```python
from build123d import *

# Parameters (mm, degrees)
CROQUIS1_W              = 480
CROQUIS1_H              = 310
CROQUIS1_W_2            = 28
CROQUIS1_H_2            = 12
CROQUIS1_H_3            = 11
CROQUIS1_W_3            = 41.3
CROQUIS1_H_4            = 41.3
SALIENTE_EXTRUIR1_DEPTH = 12
SKETCH1_R               = 1.5
CUT_EXTRUDE1_DEPTH      = 572.527777103
SKETCH2_R               = 1.55
CUT_EXTRUDE2_DEPTH      = 12
FILLET1_R               = 5
SKETCH3_R               = 1.55
CUT_EXTRUDE3_DEPTH      = 12
BOSS_EXTRUDE1_DEPTH     = 12
FILLET2_R               = 5


with BuildPart() as part:
    # Croquis1 → Saliente-Extruir1 (new body)
    with BuildSketch(Plane(origin=(0, 0, 0), x_dir=(0, 0, -1), z_dir=(1, 0, 0))):
        with Locations((240, -155)):
            Rectangle(CROQUIS1_W, CROQUIS1_H)
        Polygon((30, -30), (450, -30), (450, -114.35), (388.7, -114.35), (388.7, -195.65), (450, -195.65), (450, -280), (30, -280), (30, -181), (70, -181), (70, -161), (30, -161), (30, -149), (70, -149), (70, -129), (30, -129), align=None, mode=Mode.SUBTRACT)
        with Locations((288, -295)):
            Rectangle(CROQUIS1_W_2, CROQUIS1_H_2, mode=Mode.SUBTRACT)
        with Locations((240, -294.5)):
            Rectangle(CROQUIS1_W_2, CROQUIS1_H_3, mode=Mode.SUBTRACT)
        with Locations((192, -295)):
            Rectangle(CROQUIS1_W_2, CROQUIS1_H_2, mode=Mode.SUBTRACT)
        with Locations((192, -15)):
            Rectangle(CROQUIS1_W_2, CROQUIS1_H_2, mode=Mode.SUBTRACT)
        with Locations((288, -15)):
            Rectangle(CROQUIS1_W_2, CROQUIS1_H_2, mode=Mode.SUBTRACT)
        with Locations((240, -15.5)):
            Rectangle(CROQUIS1_W_2, CROQUIS1_H_3, mode=Mode.SUBTRACT)
        with Locations((429.35, -155)):
            Rectangle(CROQUIS1_W_3, CROQUIS1_H_4, mode=Mode.SUBTRACT)
    extrude(amount=SALIENTE_EXTRUIR1_DEPTH)

    # Sketch1 → Cut-Extrude1 (cut, through all)
    with BuildSketch(Plane(origin=(12, 0, 0), x_dir=(0, 0, -1), z_dir=(1, 0, 0))):
        with Locations((204.939339828, -10.060660172)):
            Circle(SKETCH1_R)
        with Locations((179.060660172, -10.060660172)):
            Circle(SKETCH1_R)
        with Locations((227.060660172, -11.060660172)):
            Circle(SKETCH1_R)
        with Locations((227.060660172, -19.939339828)):
            Circle(SKETCH1_R)
        with Locations((252.939339828, -11.060660172)):
            Circle(SKETCH1_R)
        with Locations((252.939339828, -19.939339828)):
            Circle(SKETCH1_R)
        with Locations((275.060660172, -10.060660172)):
            Circle(SKETCH1_R)
        with Locations((275.060660172, -19.939339828)):
            Circle(SKETCH1_R)
        with Locations((300.939339828, -19.939339828)):
            Circle(SKETCH1_R)
        with Locations((300.939339828, -10.060660172)):
            Circle(SKETCH1_R)
        with Locations((409.760660172, -135.410660172)):
            Circle(SKETCH1_R)
        with Locations((448.939339828, -135.410660172)):
            Circle(SKETCH1_R)
        with Locations((448.939339828, -174.589339828)):
            Circle(SKETCH1_R)
        with Locations((409.760660172, -174.589339828)):
            Circle(SKETCH1_R)
        with Locations((179.060660172, -19.939339828)):
            Circle(SKETCH1_R)
        with Locations((204.939339828, -19.939339828)):
            Circle(SKETCH1_R)
        with Locations((204.939339828, -290.060660172)):
            Circle(SKETCH1_R)
        with Locations((179.060660172, -290.060660172)):
            Circle(SKETCH1_R)
        with Locations((300.939339828, -299.939339828)):
            Circle(SKETCH1_R)
        with Locations((300.939339828, -290.060660172)):
            Circle(SKETCH1_R)
        with Locations((275.060660172, -290.060660172)):
            Circle(SKETCH1_R)
        with Locations((275.060660172, -299.939339828)):
            Circle(SKETCH1_R)
        with Locations((252.939339828, -290.060660172)):
            Circle(SKETCH1_R)
        with Locations((252.939339828, -298.939339828)):
            Circle(SKETCH1_R)
        with Locations((227.060660172, -290.060660172)):
            Circle(SKETCH1_R)
        with Locations((227.060660172, -298.939339828)):
            Circle(SKETCH1_R)
        with Locations((179.060660172, -299.939339828)):
            Circle(SKETCH1_R)
        with Locations((204.939339828, -299.939339828)):
            Circle(SKETCH1_R)
    extrude(amount=-CUT_EXTRUDE1_DEPTH, mode=Mode.SUBTRACT)

    # Sketch2 → Cut-Extrude2 (cut)
    with BuildSketch(Plane(origin=(12, 0, 0), x_dir=(0, 0, -1), z_dir=(1, 0, 0))):
        with Locations((60, -171)):
            Circle(SKETCH2_R)
        with Locations((35, -171)):
            Circle(SKETCH2_R)
        with Locations((35, -139)):
            Circle(SKETCH2_R)
        with Locations((60, -139)):
            Circle(SKETCH2_R)
    extrude(amount=-CUT_EXTRUDE2_DEPTH, mode=Mode.SUBTRACT)

    # Fillet1
    fillet1_edges = [part.edges().sort_by_distance(p)[0] for p in [
        (6, -30, -30),
        (6, -129, -70),
        (6, -149, -70),
        (6, -149, -30),
        (6, -161, -30),
        (6, -161, -70),
        (6, -181, -70),
        (6, -280, -30),
        (6, -280, -450),
        (6, -195.65, -388.7),
        (6, -114.35, -388.7),
        (6, -30, -450),
    ]]
    fillet(fillet1_edges, radius=FILLET1_R)

    # Sketch3 → Cut-Extrude3 (cut)
    with BuildSketch(Plane(origin=(12, 0, 0), x_dir=(0, 0, -1), z_dir=(1, 0, 0))):
        with Locations((427.52464912, -185.65)):
            Circle(SKETCH3_R)
        with Locations((460, -153.912701142)):
            Circle(SKETCH3_R)
        with Locations((427.52464912, -124.35)):
            Circle(SKETCH3_R)
        with Locations((398.7, -153.912701142)):
            Circle(SKETCH3_R)
    extrude(amount=-CUT_EXTRUDE3_DEPTH, mode=Mode.SUBTRACT)

    # Sketch4 → Boss-Extrude1 (add)
    with BuildSketch(Plane(origin=(12, 0, 0), x_dir=(0, 0, -1), z_dir=(1, 0, 0))):
        Polygon((421.85, -114.35), (450, -74.675), (450, -114.35), align=None)
        Polygon((421.85, -195.65), (450, -235.325), (450, -195.65), align=None)
        Polygon((47.5, -129), (30, -82), (30, -129), align=None)
        Polygon((47.5, -181), (30, -228), (30, -181), align=None)
    extrude(amount=-BOSS_EXTRUDE1_DEPTH)

    # Fillet2
    fillet2_edges = [part.edges().sort_by_distance(p)[0] for p in [
        (6, -114.35, -421.85),
        (6, -74.675, -450),
        (6, -195.65, -421.85),
        (6, -235.325, -450),
        (6, -129, -47.5),
        (6, -82, -30),
        (6, -181, -47.5),
        (6, -228, -30),
    ]]
    fillet(fillet2_edges, radius=FILLET2_R)


solid = part.part
```
Could you check a few things on this model? Use its own coordinates, in mm. Round coordinates to 2 decimals unless told otherwise and drop trailing zeros. Loops run counter-clockwise (first coordinate to the right, second up) from the corner with the lowest first, then second, coordinate; pieces in that order, holes last. Notation, with made-up numbers: M 13.5,-23 L 56.5,-23 A32 cw 56.5,5 Z; hole C -22,16 d11. An arc over 180 degrees is marked long. Answer as CSV lines item,"result".
1) Imagine slicing it at D-D on x = 6.5. Count the separate pieces of the cut face and the enclosed holes in it, and give its area (3 significant figures).
From the geometry:
separate pieces,"1"
enclosed holes,"16"
area,"48,600 mm^2"
2) Imagine slicing it at B-B on z = -188. List the corners of the cut face in (x, y) for me.
From the geometry:
outline,"M 0,-310 L 12,-310 L 12,-301 L 0,-301 Z; M 0,-289 L 12,-289 L 12,-280 L 0,-280 Z; M 0,-30 L 12,-30 L 12,-21 L 0,-21 Z; M 0,-9 L 12,-9 L 12,0 L 0,0 Z"
3) If I drill on probe 1 along Y at (x, z) = (6, -230); probe 2 along Z at (x, y) = (8.5, -139); probe 3 along Z at (x, y) = (5.75, -142.5), over which ranges is the centre line in solid material (lowest first)?
From the geometry:
probe 1,"-310 to -300, -289 to -280, -30 to -21, -10 to 0"
probe 2,"-480 to -450, -408.7 to -388.7, -70 to -61.55, -58.45 to -36.55, -33.45 to 0"
probe 3,"-480 to -450, -408.7 to -388.7, -70 to 0"
4) Imagine slicing it at C-C on y = -269. List the corners of the cut face in (x, z) for me, and give its area (3 significant figures).
From the geometry:
outline,"M 0,-480 L 12,-480 L 12,-450 L 0,-450 Z; M 0,-30 L 12,-30 L 12,0 L 0,0 Z"
area,"720 mm^2"
5) Imagine slicing it at A-A on z = -368. List the corners of the cut face in (x, y) for me, and give its area (3 significant figures).
From the geometry:
outline,"M 0,-310 L 12,-310 L 12,-280 L 0,-280 Z; M 0,-30 L 12,-30 L 12,0 L 0,0 Z"
area,"720 mm^2"
6) We'd pull the mould along Z, two halves only. Please class faces 1 (the flat face through (0, -28, -259)), 2 (the flat face through (6.084, -215.637, -436.031)): released by +Z, released by -Z, zero draft, split by the parting line, or undercut.
From the geometry:
face 1,"zero draft"
face 2,"undercut"
